Here's the drawing with two shaded views (mm, measured from the low corner). I have some questions. Give positions to 0.01 mm unless a question says otherwise; leave off trailing zeros. Write each loop counter-clockwise with the first axis right and the second up, starting at its lowest first coordinate (ties: lowest second). Pieces come first, ordered by that corner, then holes.
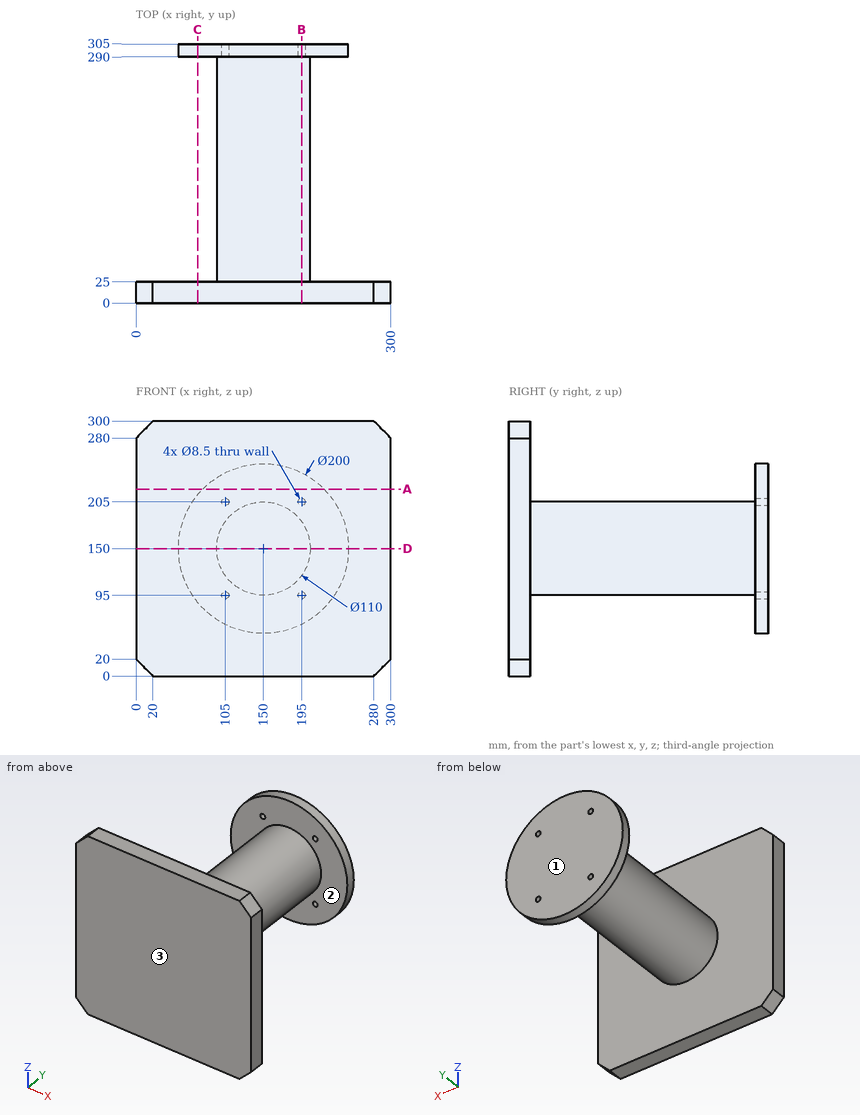
(1) Imagine slicing it at D-D, the plane z = 150. Write out the boundary of the cut face in (x, y).
Returned:
outline: (0, 0) - (300, 0) - (300, 25) - (205, 25) - (205, 290) - (250, 290) - (250, 305) - (50, 305) - (50, 290) - (95, 290) - (95, 25) - (0, 25) - close
(2) Imagine slicing it at C-C, the plane x = 72.5. Write out the boundary of the cut face in (y, z).
Returned:
outline: (0, 0) - (25, 0) - (25, 300) - (0, 300) - close; (290, 86.8) - (305, 86.8) - (305, 213.2) - (290, 213.2) - close
(3) Imagine slicing it at A-A, the plane z = 220. Write out the boundary of the cut face in (x, y), plus the area to 3 significant figures.
Returned:
outline: (0, 0) - (300, 0) - (300, 25) - (0, 25) - close; (78.59, 290) - (221.41, 290) - (221.41, 305) - (78.59, 305) - close
area: 9,640 mm2
(4) If I drill on L1, parallel to Y at x = 153, z = 207; L2, parallel to X at y = 297.75, z = 205; L3, parallel to Z at x = 105, y = 296, over which ranges is the centre line in solid material (lowest first)?
Returned:
L1: y = 0 to 25, 290 to 305
L2: x = 66.48 to 100.75, 109.25 to 190.75, 199.25 to 233.52
L3: z = 60.7 to 90.75, 99.25 to 200.75, 209.25 to 239.3
(5) Will these pins go through, and if not, where does the flat tip stop? P1, Ø7.5, axis at x = 195, z = 95, coming from the -Y side; P2, Ø1.5, axis at x = 189.5, y = 134, coming from the -Z side; P3, Ø2, axis at x = 258, z = 269.5, coming from the +Y side; P4, Ø10, axis at y = 48, z = 108.5, coming from the +X side.
Returned:
P1: stops at y = 0
P2: stops at z = 110.97
P3: stops at y = 25
P4: stops at x = 191.14
(6) If we mould it in two halves opening along Y, with no side actions, what happens to the marked faces 1, 2 and 3? For each: +Y half, -Y half, draft (parallel to the pull), parting line (faces both ways), or undercut.
Returned:
face 1: +Y half
face 2: undercut
face 3: -Y half
(7) Imagine slicing it at B-B, the plane x = 195. Write out the boundary of the cut face in (y, z), plus the area to 3 significant figures.
Returned:
outline: (0, 0) - (25, 0) - (25, 118.38) - (290, 118.38) - (290, 99.25) - (305, 99.25) - (305, 200.75) - (290, 200.75) - (290, 181.62) - (25, 181.62) - (25, 300) - (0, 300) - close; (290, 60.7) - (305, 60.7) - (305, 90.75) - (290, 90.75) - close; (290, 209.25) - (305, 209.25) - (305, 239.3) - (290, 239.3) - close
area: 26,700 mm2
